Check sheet for the drawn part. Datum: minimum x, y, z corner. Units: mm. Coordinates: 2 decimals unless noted, no trailing zeros. Order: outer loops, then holes, each group sorted by start corner. A loop starts at its lowest first (then second) coordinate and runs counter-clockwise, first axis right, second up. Notation, with made-up numbers: M 86,58 L 125,58 A23 ccw 125,72 Z; hole C 87.5,46.5 d3. An arc over 180 degrees is marked long. Use one line per item in the form item = value. Start each with the question number.
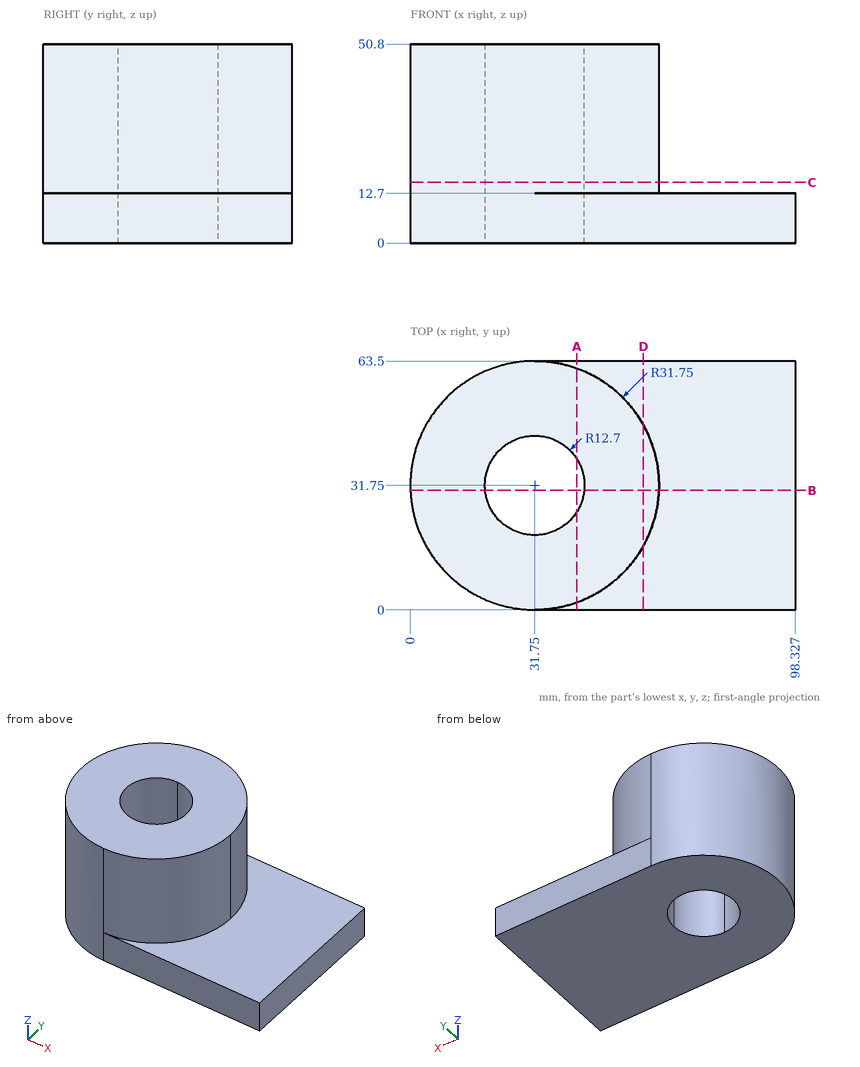
1. Depth check by flat-ended pin: P1, Ø3, axis at y = 34.5, z = 22.5, coming from the +X side; P2, Ø8, axis at y = 11, z = 32.5, coming from the -X side; P3, Ø1.5, axis at x = 83, y = 37.5, coming from the +Z side. Enter the tip coordinate at first touch or a pass-through.
2. Cross-section at B-B on y = 30.5. Enter the section's corners in (x, z) (1 decimal).
3. Material ranges on line 1 along Y through (x, z) = (32.5, 15); line 2 along Z through (x, y) = (68.5, 59); line 3 along X through (y, z) = (40, 22) (1 decimal), recorded low to high.
4. Cross-section at D-D on x = 59.5. Enter the section's corners in (y, z).
5. Cross-section at C-C on z = 15.5. Enter the section's corners in (x, y).
6. Cross-section at A-A on x = 42.5. Enter the section's corners in (y, z) (1 decimal).
Final values:
q1.P1 = 63.48
q1.P2 = 4.78
q1.P3 = 12.7
q2.outline = M 0,0 L 19.1,0 L 19.1,50.8 L 0,50.8 Z; M 44.4,0 L 98.3,0 L 98.3,12.7 L 63.5,12.7 L 63.5,50.8 L 44.4,50.8 Z
q3.line_1 = 0.01 to 19.07, 44.43 to 63.49
q3.line_2 = 0 to 12.7
q3.line_3 = 1.1 to 22.1, 41.4 to 62.4
q4.outline = M 0,0 L 63.5,0 L 63.5,12.7 L 47.18,12.7 L 47.18,50.8 L 16.32,50.8 L 16.32,12.7 L 0,12.7 Z
q5.outline = M 31.75,0 A31.75 ccw 63.5,31.75 A31.75 ccw 31.75,63.5 A31.75 ccw Z; hole C 31.75,31.75 d25.4
q6.outline = M 0,0 L 25,0 L 25,50.8 L 1.9,50.8 L 1.9,12.7 L 0,12.7 Z; M 38.5,0 L 63.5,0 L 63.5,12.7 L 61.6,12.7 L 61.6,50.8 L 38.5,50.8 Z
